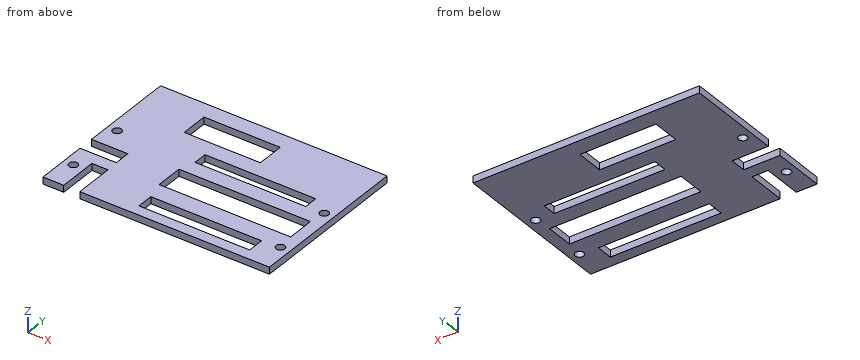
```python
from build123d import *

# Parameters (mm, degrees)
F0_R     = 1.9812
F0_W     = 50.8
F0_H     = 7.62
F0_W_2   = 60.325
F0_H_2   = 12.7
F0_W_3   = 34.925
F0_H_3   = 6.35
F1_DEPTH = 3.175


with BuildPart() as f1:
    # F0 (on Top) → F1 (new body)
    with BuildSketch(Plane.XY):
        Polygon((0, 23.7363), (0, 0), (9.51992, 0), (9.51992, 18.034), (16.88592, 18.034), (16.88592, 0), (103.886, 0), (103.886, 75.2983), (0, 75.2983), (0, 31.1023), (16.64462, 31.1023), (16.64462, 23.7363), align=None)
        with Locations((4.445, 13.2842)):
            Circle(F0_R, mode=Mode.SUBTRACT)
        with Locations((65.786, 8.89)):
            Rectangle(F0_W, F0_H, mode=Mode.SUBTRACT)
        with Locations((99.441, 13.27912)):
            Circle(F0_R, mode=Mode.SUBTRACT)
        with Locations((68.326, 27.432)):
            Rectangle(F0_W_2, F0_H_2, mode=Mode.SUBTRACT)
        with Locations((4.445, 41.3131)):
            Circle(F0_R, mode=Mode.SUBTRACT)
        with Locations((42.8625, 61.3283)):
            Rectangle(F0_W_3, F0_H_2, mode=Mode.SUBTRACT)
        with Locations((65.786, 44.1833)):
            Rectangle(F0_W, F0_H_3, mode=Mode.SUBTRACT)
        with Locations((99.441, 41.3131)):
            Circle(F0_R, mode=Mode.SUBTRACT)
    extrude(amount=F1_DEPTH)


solid = f1.part
```
Here's how the part is built. I have some questions about the finished solid (model axes, mm). Round coordinates to 2 decimals unless told otherwise and drop trailing zeros. Loops run counter-clockwise (first coordinate to the right, second up) from the corner with the lowest first, then second, coordinate; pieces in that order, holes last. Notation, with made-up numbers: (33, 47) -> (49, 47) arc R21 cw to (49, 56) -> close; hole circle Ø5 at (-24.75, -28.75). An arc over 180 degrees is marked (long way). Answer as CSV lines item,"result". Start each with the question number.
1. I'm going to push a flat-ended pin straight in: P1, Ø5, axis at x = 99.44, y = 13.28, coming from the +Z side (3 decimals). Where does the tip first touch, or does it pass through?
2. Imagine slicing it at A-A on x = 55. Write out the boundary of the cut face in (y, z) (3 decimals), plus the area to 3 significant figures.
3. I need wall thicknesses on probe 1 along Y at (x, z) = (50.5, 0.4); probe 2 along Y at (x, z) = (77, 2.1); probe 3 along X at (y, z) = (11, 0.2). Which ranges of each line are inside material? Lowest first, please. Write a range as from..to.
4. Imagine slicing it at B-B on x = 8. Write out the boundary of the cut face in (y, z) (3 decimals), plus the area to 3 significant figures.
5. Imagine slicing it at C-C on z = 1.7. State how many separate pieces and enclosed holes the cut face has, plus the area to 3 significant figures.
Solution:
1,P1,"z = 3.175"
2,outline,"(0, 0) -> (5.08, 0) -> (5.08, 3.175) -> (0, 3.175) -> close; (12.7, 0) -> (21.082, 0) -> (21.082, 3.175) -> (12.7, 3.175) -> close; (33.782, 0) -> (41.008, 0) -> (41.008, 3.175) -> (33.782, 3.175) -> close; (47.358, 0) -> (54.978, 0) -> (54.978, 3.175) -> (47.358, 3.175) -> close; (67.678, 0) -> (75.298, 0) -> (75.298, 3.175) -> (67.678, 3.175) -> close"
2,area,"114 mm²"
3,probe 1,"0..5.08, 12.7..21.08, 33.78..41.01, 47.36..54.98, 67.68..75.3"
3,probe 2,"0..5.08, 12.7..21.08, 33.78..41.01, 47.36..75.3"
3,probe 3,"0..9.52, 16.89..40.39, 91.19..103.89"
4,outline,"(0, 0) -> (23.736, 0) -> (23.736, 3.175) -> (0, 3.175) -> close; (31.102, 0) -> (75.298, 0) -> (75.298, 3.175) -> (31.102, 3.175) -> close"
4,area,"216 mm²"
5,separate pieces,"1"
5,enclosed holes,"8"
5,area,"5,600 mm²"
